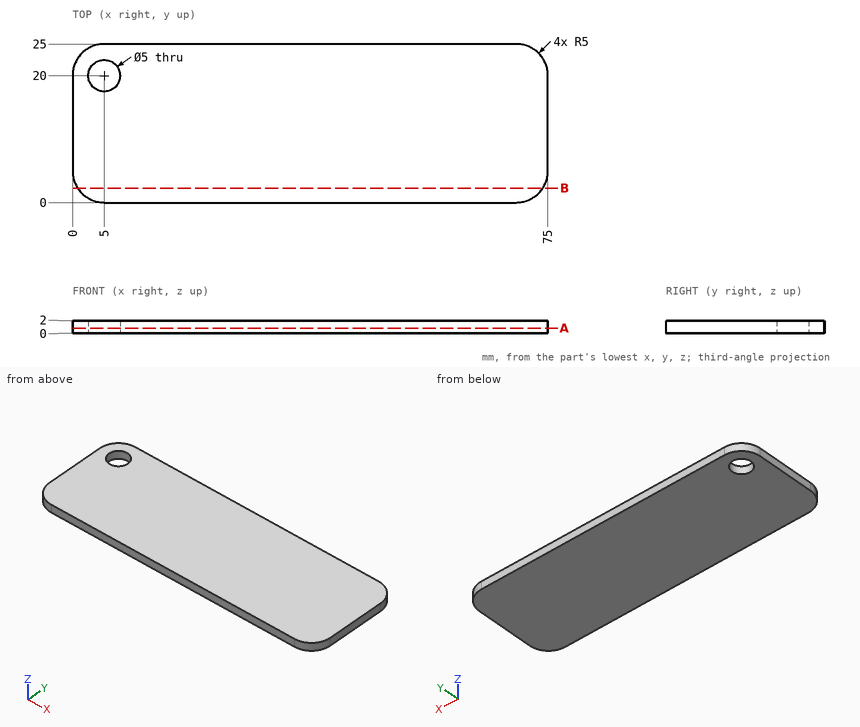
Part print with two shaded views. Sizes in mm from the minimum x, y, z corner. Give positions to 0.01 mm unless a question says otherwise; leave off trailing zeros. Order: outer loops, then holes, each group sorted by start corner. A loop starts at its lowest first (then second) coordinate and runs counter-clockwise, first axis right, second up.
(1) Flat gauge pins, fed straight in: pin 1 (6 mm diameter, centred on x = 53, y = 8.5, fed in from -Z); pin 2 (3 mm diameter, centred on x = 5, y = 20, fed in from -Z). Where does each tip first touch, or does it go through?
(2) Saw through at B-B, the plane y = 2.25. Give the cut face in (x, z).
(3) Saw through at A-A, the plane z = 0.8. Give the cut face in (x, y).
(4) Drill centre lines: L1, parallel to X at y = 19.5, z = 0.8; L2, parallel to Y at x = 4.5, z = 1.3; L3, parallel to X at y = 18.5, z = 1.85. Where is each one in solid material? Low to high.
Results found:
1. pin 1: stops at z = 0
1. pin 2: passes through
2. outline: (0.82, 0) - (74.18, 0) - (74.18, 2) - (0.82, 2) - close
3. outline: (0, 5) arc R5 ccw to (5, 0) - (70, 0) arc R5 ccw to (75, 5) - (75, 20) arc R5 ccw to (70, 25) - (5, 25) arc R5 ccw to (0, 20) - close; hole circle Ø5 at (5, 20)
4. L1: x = 0 to 2.55, 7.45 to 75
4. L2: y = 0.03 to 17.55, 22.45 to 24.97
4. L3: x = 0 to 3, 7 to 75
